```python
from build123d import *

# Parameters (mm, degrees)
F0_W     = 19.05
F0_H     = 314.1864430949
F1_DEPTH = 381
F2_W     = 352.679
F2_H     = 31.75
F3_DEPTH = 184.15


with BuildPart() as f1:
    # F0 (on Front) → F1 (new body, symmetric)
    with BuildSketch(Plane.XZ):
        Polygon((-184.15, 0), (0, 0), (184.15, 0), (184.15, 31.75), (165.1, 31.75), (146.05, 31.75), (-146.05, 31.75), (-165.1, 31.75), (-184.15, 31.75), align=None)
        with Locations((155.575, 188.8432215475)):
            Rectangle(F0_W, F0_H)
        with Locations((-155.575, 188.8432215475)):
            Rectangle(F0_W, F0_H)
    extrude(amount=F1_DEPTH, both=True)

    # F2 (on Right) → F3 (cut, symmetric)
    with BuildSketch(Plane.YZ):
        with Locations((0, 15.875)):
            Rectangle(F2_W, F2_H)
    extrude(amount=F3_DEPTH, both=True, mode=Mode.SUBTRACT)


solid = f1.part
```
CAD build for the part. Positions are in the model's coordinates, mm. A direction names the side the tool comes from. Round coordinates to 2 decimals unless told otherwise and drop trailing zeros. Order: outer loops, then holes, each group sorted by start corner. A loop starts at its lowest first (then second) coordinate and runs counter-clockwise, first axis right, second up. Notation, with made-up numbers: (-6.5, -32) -> (3.5, -32) arc R12 ccw to (3.5, -22) -> close; hole circle Ø8 at (71, -30.5). An arc over 180 degrees is marked (long way). One line per question, with ' | ' between items.
Q1. Slice it at A-A (y = -157). Write the cut outline in (x, z).
Completed:
outline: (-165.1, 31.75) -> (-146.05, 31.75) -> (-146.05, 345.94) -> (-165.1, 345.94) -> close; (146.05, 31.75) -> (165.1, 31.75) -> (165.1, 345.94) -> (146.05, 345.94) -> close
Q2. Drop flat-ended pins along their axis: pin 1 (5.5 mm diameter, centred on x = 159, y = -51.5, fed in from -Z); pin 2 (1.5 mm diameter, centred on y = -65, z = 229, fed in from -X); pin 3 (21 mm diameter, centred on x = -176, y = -277, fed in from +Z); pin 4 (3 mm diameter, centred on x = -77, y = 289, fed in from -Z). Give the stop position or say it passes through.
Completed:
pin 1: stops at z = 31.75 | pin 2: stops at x = -165.1 | pin 3: stops at z = 31.75 | pin 4: stops at z = 0
Q3. Which spindle directions (+Z, -Z, +X, -X, +Y, -Y) get a long thin tool onto all of the face, cutting with end or side? Do faces 1 (the flat face through (-155, -2, 31.75)), 2 (the flat face through (-146.05, -5, 187)), 3 (the flat face through (-174, -280, 31.75)). Say none if no direction does.
Completed:
face 1: -Z, +X, -X | face 2: +Z, +Y, -Y | face 3: +Z, -X, +Y, -Y
Q4. Two-plate mould, pull along X, no slides. Class faces 4 (the flat face through (3, 176.34, 16)), 5 (the flat face through (184.15, -280, 16)), 6 (the flat face through (2, 277, 31.75)): released by +X, released by -X, zero draft, split by the parting line, or undercut.
Completed:
face 4: zero draft | face 5: released by +X | face 6: undercut
Q5. Slice it at B-B (z = 23). Write the cut outline in (x, y).
Completed:
outline: (-184.15, -381) -> (184.15, -381) -> (184.15, -176.34) -> (-184.15, -176.34) -> close; (-184.15, 176.34) -> (184.15, 176.34) -> (184.15, 381) -> (-184.15, 381) -> close
Q6. Probe probe 1 along X at (y, z) = (300.5, 40); probe 2 along Y at (x, z) = (142, 29.5); probe 3 along Z at (x, y) = (93.5, -327). List the from-to ranges inside material, lowest first.
Completed:
probe 1: x = -165.1 to -146.05, 146.05 to 165.1 | probe 2: y = -381 to -176.34, 176.34 to 381 | probe 3: z = 0 to 31.75
Q7. Slice it at C-C (y = 312.5). Write the cut outline in (x, z).
Completed:
outline: (-184.15, 0) -> (184.15, 0) -> (184.15, 31.75) -> (165.1, 31.75) -> (165.1, 345.94) -> (146.05, 345.94) -> (146.05, 31.75) -> (-146.05, 31.75) -> (-146.05, 345.94) -> (-165.1, 345.94) -> (-165.1, 31.75) -> (-184.15, 31.75) -> close
